from build123d import *

# Parameters (mm, degrees)
SKETCH1_W           = 22.098
SKETCH1_H           = 19.939
SKETCH1_R           = 1.5748
SKETCH1_R_2         = 0.4826
BOSS_EXTRUDE1_DEPTH = 1.6002
SKETCH2_W           = 7.874
SKETCH2_H           = 7.7216
BOSS_EXTRUDE2_DEPTH = 9.3472
SKETCH7_R           = 8.1915
BOSS_EXTRUDE6_DEPTH = 13.6398
SKETCH8_W           = 4.572
SKETCH8_H           = 6.604
BOSS_EXTRUDE7_DEPTH = 2.032
FILLET2_R           = 0.508
FILLET3_R           = 0.508


with BuildPart() as part:
    # Sketch1 → Boss-Extrude1 (new body)
    with BuildSketch(Plane(origin=(0, 0, 0), x_dir=(1, 0, 0), z_dir=(0, 1, 0))):
        Rectangle(SKETCH1_W, SKETCH1_H)
        with Locations(Location((8.509, 7.4295, 0), (0, 0, 270))):
            Circle(SKETCH1_R, mode=Mode.SUBTRACT)
        with Locations(Location((-8.509, -5.5245, 0), (0, 0, 270))):
            Circle(SKETCH1_R, mode=Mode.SUBTRACT)
        with Locations(Location((9.398, -8.6995, 0), (0, 0, 270))):
            Circle(SKETCH1_R_2, mode=Mode.SUBTRACT)
        with Locations(Location((6.858, -8.6995, 0), (0, 0, 270))):
            Circle(SKETCH1_R_2, mode=Mode.SUBTRACT)
        with Locations(Location((4.318, -8.6995, 0), (0, 0, 270))):
            Circle(SKETCH1_R_2, mode=Mode.SUBTRACT)
        with Locations(Location((1.778, -8.6995, 0), (0, 0, 270))):
            Circle(SKETCH1_R_2, mode=Mode.SUBTRACT)
        with Locations(Location((-0.762, -8.6995, 0), (0, 0, 270))):
            Circle(SKETCH1_R_2, mode=Mode.SUBTRACT)
        with Locations(Location((-3.302, -8.6995, 0), (0, 0, 270))):
            Circle(SKETCH1_R_2, mode=Mode.SUBTRACT)
        with Locations(Location((-5.842, -8.6995, 0), (0, 0, 270))):
            Circle(SKETCH1_R_2, mode=Mode.SUBTRACT)
    extrude(amount=BOSS_EXTRUDE1_DEPTH)

    # Sketch2 → Boss-Extrude2 (add)
    with BuildSketch(Plane(origin=(0, 1.6002, 0), x_dir=(1, 0, 0), z_dir=(0, 1, 0))):
        with Locations((5.3848, -2.8067)):
            Rectangle(SKETCH2_W, SKETCH2_H)
    extrude(amount=BOSS_EXTRUDE2_DEPTH)

    # Sketch7 → Boss-Extrude6 (add)
    with BuildSketch(Plane.XZ):
        with Locations(Location((0, -0.5207, 0), (0, 0, 270))):
            Circle(SKETCH7_R)
    extrude(amount=BOSS_EXTRUDE6_DEPTH)

    # Sketch8 → Boss-Extrude7 (add)
    with BuildSketch(Plane.XZ):
        with Locations((-8.255, -4.6355)):
            Rectangle(SKETCH8_W, SKETCH8_H)
    extrude(amount=BOSS_EXTRUDE7_DEPTH)

    # Fillet2
    fillet2_edges = [part.edges().sort_by_distance(p)[0] for p in [
        (0, -13.6398, 7.6708),
    ]]
    fillet(fillet2_edges, radius=FILLET2_R)

    # Fillet3
    fillet3_edges = [part.edges().sort_by_distance(p)[0] for p in [
        (1.4478, 10.9474, 2.8067),
        (5.3848, 10.9474, 6.6675),
        (9.3218, 10.9474, 2.8067),
        (5.3848, 10.9474, -1.0541),
    ]]
    fillet(fillet3_edges, radius=FILLET3_R)


solid = part.part
Could you check a few things on this model? Use its own coordinates, in mm. A direction names the side the tool comes from. Give positions to 0.01 mm unless a question says otherwise; leave off trailing zeros. Write each loop counter-clockwise with the first axis right and the second up, starting at its lowest first coordinate (ties: lowest second). Pieces come first, ordered by that corner, then holes. Notation, with made-up numbers: (53, -12.5) -> (58, -12.5) arc R27 ccw to (58, 7.5) -> close; hole circle Ø11 at (52.5, -21.5). An arc over 180 degrees is marked (long way). Answer as CSV lines item,"result". Start each with the question number.
(1) Please list where these lines run through material, in increasing order: line 1 (Y direction, x = -3.5, z = -1.25); line 2 (X direction, y = 2.5, z = 1.5); line 3 (Z direction, x = 7, y = 6.5).
(2) If we section it at A-A, the plane y = 6: Write out the boundary of the cut face in (x, z), and give its area (3 significant figures).
(3) If we mould it in two halves opening along X, with no side actions, what happens to faces 1 (the face through (1.448, 6, 3)), 2 (the face through (-9, -1, -1.334)), 3 (the face through (8.93, 0.79, 8.59)), 4 (the face through (6.39, 0.79, 8.59))? For each: +X half, -X half, draft (parallel to the pull), parting line (faces both ways), or undercut.
(4) I'm going to push flat-ended pins straight in: pin 1 Ø6 at (y, z) = (7, 2) entering from -X; pin 2 Ø2 at (x, y) = (6, -9.5) entering from +Z; pin 3 Ø1 at (x, y) = (7.5, -5.5) entering from +Z. Where does each tip first touch, or does it pass through?
(5) Which directions (+Z, -Z, +X, -X, +Y, -Y) give clear straight access to the entire face, cutting with the end or side of a thin tool? Please do faces 5 (the face through (-9, -2.032, -5)), 6 (the face through (5, 6, -1.054)), 7 (the face through (8.12, -6.47, 0.55)), 8 (the face through (-10.541, -1, -5)).
(6) If we section it at B-B, the plane y = -11.5: Write out the boundary of the cut face in (x, z), and give its area (3 significant figures).
Answer list:
1,line 1,"-13.64 to 1.6"
1,line 2,"1.45 to 9.32"
1,line 3,"-1.05 to 6.67"
2,outline,"(1.45, -1.05) -> (9.32, -1.05) -> (9.32, 6.67) -> (1.45, 6.67) -> close"
2,area,"60.8 mm^2"
3,face 1,"-X half"
3,face 2,"draft"
3,face 3,"undercut"
3,face 4,"undercut"
4,pin 1,"x = 1.45"
4,pin 2,"z = 5.97"
4,pin 3,"z = 3.73"
5,face 5,"-Z, -X, -Y"
5,face 6,"-Z, +X, -X, +Y"
5,face 7,"-Y"
5,face 8,"+Z, -Z, -X, -Y"
6,outline,"circle Ø16.38 at (0, -0.52)"
6,area,"211 mm^2"
